Could you check a few things on this model? Use its own coordinates, in mm. A direction names the side the tool comes from. Give positions to 0.01 mm unless a question says otherwise; leave off trailing zeros. Loops run counter-clockwise (first coordinate to the right, second up) from the corner with the lowest first, then second, coordinate; pieces in that order, holes last. Notation, with made-up numbers: (65.5, 2) -> (124.5, 2) arc R34 cw to (124.5, 32) -> close; hole circle Ø11 at (-19.5, 66.5). An arc over 180 degrees is marked (long way). Put each result on its own line as item: value.
Autodesk Inventor part; units mm, degrees
ref_plane "YZ Plane" through (0, 0, 0) normal (1, 0, 0) x (0, 1, 0)
ref_plane "XZ Plane" through (0, 0, 0) normal (0, 1, 0) x (-1, 0, 0)
ref_plane "XY Plane" through (0, 0, 0) normal (0, 0, 1) x (1, 0, 0)
sketch "Sketch1" plane through (0, 0, 0) normal (0, 1, 0) x (-1, 0, 0)
  line L0 (0.5774, -1) -> (8.6603, -15)
  line L1 (8.6603, -15) -> (6.0622, -16.5)
  line L2 (-1.1547, 0) -> (-14.4338, 0)
  line L3 (-14.4338, 0) -> (-14.4338, -3)
  line L4 (-14.4338, -3) -> (-1.7898, -3)
  line L5 (-1.7032, -3.05) -> (6.0622, -16.5)
  line L6 (0, 0) -> (-8.1844, -14.1757) construction
  arc A0 (-1.7032, -3.05) -> (-1.7898, -3) centre (-1.7898, -3.1) ccw
  arc A1 (0.5774, -1) -> (-1.1547, 0) centre (-1.1547, -2) ccw
  line L7 (-19.0526, 0) -> (13.2791, 0)
  point P0 (-1.7321, -3)
  dimension "d4" = 3
  dimension "d8" = 0.1
  dimension "d9" = 2
  dimension "d16" = 120
  dimension "d19" = 12.5
  dimension "d20" = 15
extrude "Extrusion1" add sketch "Sketch1" along normal blind 15
sketch "Sketch2" plane through (0, 15, 0) normal (0, 1, 0) x (1, 0, 0)
  line L0 (-8.6603, 15) -> (-0.5774, 1)
  line L1 (1.1547, 0) -> (14.4338, 0)
  line L2 (14.4338, 0) -> (14.4338, 3)
  line L3 (14.4338, 3) -> (1.7898, 3)
  line L4 (1.7032, 3.05) -> (-6.0622, 16.5)
  line L5 (-6.0622, 16.5) -> (-8.6603, 15)
  line L6 (14.4338, 3) -> (-6.0622, 16.5)
  arc A0 (-0.5774, 1) -> (1.1547, 0) centre (1.1547, 2) ccw
  arc A1 (1.7032, 3.05) -> (1.7898, 3) centre (1.7898, 3.1) ccw
  point P0 (0, 0)
extrude "Extrusion2" add sketch "Sketch2" along normal blind 3
sketch "Sketch3" plane through (14.4338, 0, -3) normal (0, 0, -1) x (-1, 0, 0)
  line L0 (0, 0) -> (12.644, 0)
  line L1 (0, 0) -> (0, 15)
  circle A0 centre (6.322, 7.5) radius 2.25
  line L2 (12.644, 0) -> (12.644, 15)
  line L3 (0, 15) -> (12.644, 15)
  point P0 (14.4338, 0)
  point P1 (6.322, 0)
  point P2 (0, 7.5)
  dimension "d5" = 4.5
extrude "Extrusion3" cut sketch "Sketch3" against normal through all contours A0
sketch "Sketch5" plane through (-6.0622, 0, -16.5) normal (0.866, 0, -0.5) x (-0.5, 0, -0.866)
  circle A0 centre (-4.5, 7.5) radius 1.5
  line L0 (-15.5307, 0) -> (0, 0)
  line L1 (0, 0) -> (0, 15)
  line L2 (-15.5307, 15) -> (0, 15)
  line L3 (-15.5307, 0) -> (-15.5307, 15)
  point P0 (-17.3205, 0)
  point P1 (0, 7.5)
  dimension "d12" = 3
  dimension "d18" = 4.5
extrude "Extrusion4" cut sketch "Sketch5" against normal through all contours A0
fillet "Fillet1" radius 1.5 2 edges at (-7.3612, 0, -15.75) (14.4338, 0, -1.5)
properties part number "EE_adapter"
1. I need wall thicknesses on line 1 (Z direction, x = 13.25, y = 1.25); line 2 (Y direction, x = 5.5, z = -4.5); line 3 (Y direction, x = -7.5, z = -14). Which ranges of each line are inside material? Lowest first, please.
Recorded:
line 1: z = -3 to 0
line 2: y = 15 to 18
line 3: y = 0 to 18
2. Thinking about a two-plate mould opening in Y: for faces 1 (the face through (0, 0, -5)), 2 (the face through (-5, 6, -12)), 3 (the face through (10, 6, -3)), which applies, pulls with the +Y half, pulls with the -Y half, needs draft (parallel to the pull), parting line crosses it, or undercut?
Recorded:
face 1: pulls with the -Y half
face 2: undercut
face 3: needs draft
3. If we section it at D-D (z = -8.75): List the corners of the cut face in (x, y) for me, then the cut area to 3 significant figures.
Recorded:
outline: (-5.05, 0) -> (-1.59, 0) -> (-1.59, 15) -> (5.7, 15) -> (5.7, 18) -> (-5.05, 18) -> close
area: 84.2 mm^2
4. For faces 4 (the face through (-2.125, 7.395, -9.681)), 5 (the face through (6, 9, 0)), which set-ups out of +Z, -Z, +X, -X, +Y, -Y let a thin tool reach every point of the face, with its end or its side?
Recorded:
face 4: -Z, +X, -Y
face 5: +Z, +X, -X, +Y, -Y
5. If we section it at C-C (x = 12): List the corners of the cut face in (y, z) for me.
Recorded:
outline: (0, -3) -> (15, -3) -> (15, -4.6) -> (18, -4.6) -> (18, 0) -> (0, 0) -> close
6. If we section it at A-A (y = 7.5): List the corners of the cut face in (x, z) for me.
Recorded:
outline: (-8.66, -15) -> (-6.06, -16.5) -> (-4.56, -13.9) -> (-7.16, -12.4) -> close; (-5.66, -9.8) -> (-3.06, -11.3) -> (1.7, -3.05) arc R0.1 cw to (1.79, -3) -> (5.86, -3) -> (5.86, 0) -> (1.15, 0) arc R2 ccw to (-0.58, -1) -> close; (10.36, -3) -> (14.43, -3) -> (14.43, 0) -> (10.36, 0) -> close
7. I'm going to push flat-ended pins straight in: pin 1 (6 mm diameter, centred on x = 8.11, y = 7.5, fed in from -Z); pin 2 (2 mm diameter, centred on x = 2.5, y = 8.5, fed in from -Z); pin 3 (5 mm diameter, centred on y = 3.5, z = -4.5, fed in from -X). Where does each tip first touch, or does it pass through?
Recorded:
pin 1: stops at z = -3
pin 2: stops at z = -3.4
pin 3: stops at x = -4.04
8. If we section it at B-B (y = 14.25): List the corners of the cut face in (x, z) for me.
Recorded:
outline: (-8.66, -15) -> (-6.06, -16.5) -> (1.7, -3.05) arc R0.1 cw to (1.79, -3) -> (14.43, -3) -> (14.43, 0) -> (1.15, 0) arc R2 ccw to (-0.58, -1) -> close
